from build123d import *

# Parameters (mm, degrees)
F0_W     = 20
F0_H     = 7
F0_W_2   = 7
F0_H_2   = 7.875001
F1_DEPTH = 9
F2_DEPTH = 7.5


with BuildPart() as f1:
    # F0 (on Top) → F1 (new body)
    with BuildSketch(Plane.XY):
        Polygon((-39.375005, 7.875001), (-39.375005, 0), (45.783415, 0), (45.783415, 18.708905), (38.187098, 18.708905), (31.187098, 18.708905), (-27.343754, 18.708905), (-34.343754, 18.708905), (-39.375005, 18.708905), align=None)
        with Locations((-20.899706, 9.230794)):
            Rectangle(F0_W, F0_H, mode=Mode.SUBTRACT)
        with Locations((-42.875005, 3.9375)):
            Rectangle(F0_W_2, F0_H_2)
        with Locations((34.687098, 22.208905)):
            Rectangle(F0_W_2, F0_H)
        with Locations((-30.843754, 22.208905)):
            Rectangle(F0_W_2, F0_H)
        with Locations((-20.899706, 9.230794)):
            Rectangle(F0_W, F0_H)
    extrude(amount=F1_DEPTH)

    # F0 (on Top) → F2 (cut)
    with BuildSketch(Plane.XY):
        with Locations((-20.899706, 9.230794)):
            Rectangle(F0_W, F0_H)
    extrude(amount=F2_DEPTH, mode=Mode.SUBTRACT)


solid = f1.part
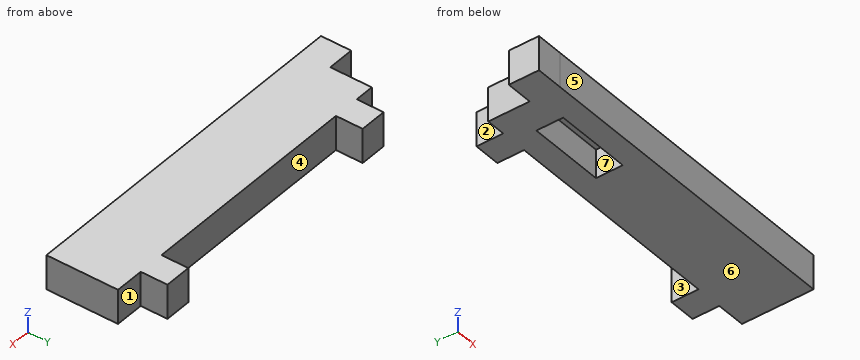
Source: CAD feature listing. Evaluate the final solid. Frame: model axes, mm. Face numbers are marked on the shaded views. A direction names the side the tool comes from. Round coordinates to 2 decimals unless told otherwise and drop trailing zeros. Order: outer loops, then holes, each group sorted by start corner. A loop starts at its lowest first (then second) coordinate and runs counter-clockwise, first axis right, second up. Notation, with made-up numbers: (41, 78.25) - (100, 78.25) arc R13 ccw to (100, 89.25) - close; hole circle Ø8 at (52.25, 19.5). An arc over 180 degrees is marked (long way). Use a Markdown table: item, result. Add a question column.
1. Set-up query: the marked faces 1, 2 and 3. Return all of +Z, -Z, +X, -X, +Y, -Y with unobstructed straight access to the full face (end or side cutting, diameter ignored); none if empty.
2. First-contact query: pin 1 (3.5 mm diameter, centred on y = 22.5, z = 2.5, fed in from -X); pin 2 (4 mm diameter, centred on x = 21.5, z = 4, fed in from +Y). Flat tips, straight axial feed; report the tip coordinate or a pass-through.
3. Section query D-D (y = 16.5). Return the cut outline in (x, z) (3 decimals).
4. Section query A-A (z = 5). Return the cut outline in (x, y) (3 decimals).
5. Section query B-B (y = 24). Return the cut outline in (x, z).
6. Section query C-C (x = -20). Return the cut outline in (y, z).
7. Line query: probe 1 along X at (y, z) = (22, 3); probe 2 along X at (y, z) = (7.75, 7) (3 decimals); probe 3 along X at (y, z) = (15.25, 0.5) (3 decimals). Output: solid intervals per line, ascending.
8. Mould query, pull axis Y, two halves, no side actions, for the marked faces 4, 5, 6 and 7. Classes: +Y half, -Y half, draft (parallel to the pull), parting line (faces both ways), or undercut.
Derived:
| question | item | result |
|---|---|---|
| 1 | face 1 | +Z, -Z, +X, +Y |
| 1 | face 2 | +Z, -Z, -X, +Y |
| 1 | face 3 | +Z, -Z, +Y |
| 2 | pin 1 | x = -34.34 |
| 2 | pin 2 | y = 18.71 |
| 3 | outline | (-39.375, 0) - (45.783, 0) - (45.783, 9) - (-39.375, 9) - close |
| 4 | outline | (-46.375, 0) - (45.783, 0) - (45.783, 18.709) - (38.187, 18.709) - (38.187, 25.709) - (31.187, 25.709) - (31.187, 18.709) - (-27.344, 18.709) - (-27.344, 25.709) - (-34.344, 25.709) - (-34.344, 18.709) - (-39.375, 18.709) - (-39.375, 7.875) - (-46.375, 7.875) - close; hole (-30.9, 5.731) - (-10.9, 5.731) - (-10.9, 12.731) - (-30.9, 12.731) - close |
| 5 | outline | (-34.34, 0) - (-27.34, 0) - (-27.34, 9) - (-34.34, 9) - close; (31.19, 0) - (38.19, 0) - (38.19, 9) - (31.19, 9) - close |
| 6 | outline | (0, 0) - (5.73, 0) - (5.73, 7.5) - (12.73, 7.5) - (12.73, 0) - (18.71, 0) - (18.71, 9) - (0, 9) - close |
| 7 | probe 1 | -34.34 to -27.34, 31.19 to 38.19 |
| 7 | probe 2 | -46.375 to -30.9, -10.9 to 45.783 |
| 7 | probe 3 | -39.375 to 45.783 |
| 8 | face 4 | +Y half |
| 8 | face 5 | -Y half |
| 8 | face 6 | draft |
| 8 | face 7 | undercut |
